Autodesk Fusion 360 part; units mm, degrees
sketch "Sketch1" plane through (0, 0, 0) normal (1, 0, 0) x (0, 1, 0)
  line L0 (0, 0) -> (0, 21)
  line L1 (0, 21) -> (5, 21)
  line L2 (5, 21) -> (5, 8)
  line L3 (5, 8) -> (35, 8)
  line L4 (35, 8) -> (35, 21)
  line L5 (35, 21) -> (40, 21)
  line L6 (40, 21) -> (40, 0)
  line L7 (40, 0) -> (0, 0)
  line L8 (20, 8) -> (20, 0) construction
  dimension "d1" = 8
  dimension "d2" = 30
  dimension "d3" = 5
  dimension "d5" = 5
  dimension "d6" = 13
  dimension "d7" = 13
extrude "Extrude1" add sketch "Sketch1" along normal blind 70
fillet "Fillet1" radius 2.5 2 edges at (35, 40, 21) (35, 0, 21)
sketch "Sketch2" plane through (0, 0, 8) normal (0, 0, 1) x (-1, 0, 0)
  line L0 (0, -35) -> (0, -5)
  line L1 (0, -5) -> (-70, -5)
  line L2 (-70, -5) -> (-70, -35)
  line L3 (-70, -35) -> (0, -35)
  line L4 (0, -5) -> (-70, -5)
  line L5 (-70, -35) -> (-70, -5)
  line L6 (0, -5) -> (0, -35)
  line L7 (0, -35) -> (-70, -35)
  line L8 (-35, -35) -> (-35, -5) construction
  line L9 (-65, -10) -> (-65, -30) construction
  line L10 (-65, -30) -> (-5, -30) construction
  line L11 (-5, -30) -> (-5, -10) construction
  line L12 (-5, -10) -> (-65, -10) construction
  line L13 (-5, -20) -> (-65, -20) construction
  line L14 (-5, -27) -> (-65, -27)
  arc A0 (-65, -27) -> (-65, -32) centre (-65, -29.5) ccw
  line L15 (-65, -32) -> (-5, -32)
  arc A1 (-5, -32) -> (-5, -27) centre (-5, -29.5) ccw
  line L16 (-5, -29.5) -> (-65, -29.5) construction
  line L17 (-65, -22.5) -> (-5, -22.5)
  arc A2 (-5, -22.5) -> (-5, -17.5) centre (-5, -20) ccw
  line L18 (-5, -17.5) -> (-65, -17.5)
  arc A3 (-65, -17.5) -> (-65, -22.5) centre (-65, -20) ccw
  line L19 (-65, -13) -> (-5, -13)
  arc A4 (-5, -13) -> (-5, -8) centre (-5, -10.5) ccw
  line L20 (-5, -8) -> (-65, -8)
  arc A5 (-65, -8) -> (-65, -13) centre (-65, -10.5) ccw
  dimension "d12" = -5
  dimension "d15" = 3
  dimension "d16" = 5
  dimension "d19" = 0
  dimension "d20" = 19
extrude "Extrude2" cut sketch "Sketch2" against normal up to surface (8 mm away) contours L14 A0 L15 A1 | L17 A2 L18 A3 | L19 A4 L20 A5
sketch "Sketch3" plane through (0, 0, 0) normal (0, -1, 0) x (1, 0, 0)
  line L0 (70, 18.5) -> (0, 18.5)
  line L1 (0, 18.5) -> (0, 0)
  line L2 (0, 0) -> (70, 0)
  line L3 (70, 0) -> (70, 18.5)
  line L4 (0, 8) -> (70, 8)
  line L5 (0, 21) -> (70, 21)
  line L6 (0, 21) -> (0, 8)
  line L7 (70, 8) -> (70, 21)
  line L8 (0, 18.5) -> (70, 18.5)
  line L9 (5.5, 10.5) -> (64.5, 10.5)
  arc A0 (64.5, 10.5) -> (64.5, 15.5) centre (64.5, 13) ccw
  line L10 (64.5, 15.5) -> (5.5, 15.5)
  arc A1 (5.5, 15.5) -> (5.5, 10.5) centre (5.5, 13) ccw
  line L11 (5.5, 13) -> (64.5, 13) construction
  dimension "d23" = 5
  dimension "d24" = 3
  dimension "d25" = 3
  dimension "d26" = 3
extrude "Extrude3" cut sketch "Sketch3" against normal up to surface (40 mm away) contours L9 A0 L10 A1
fillet "Fillet2" radius 5 2 edges at (35, 40, 0) (35, 0, 0)
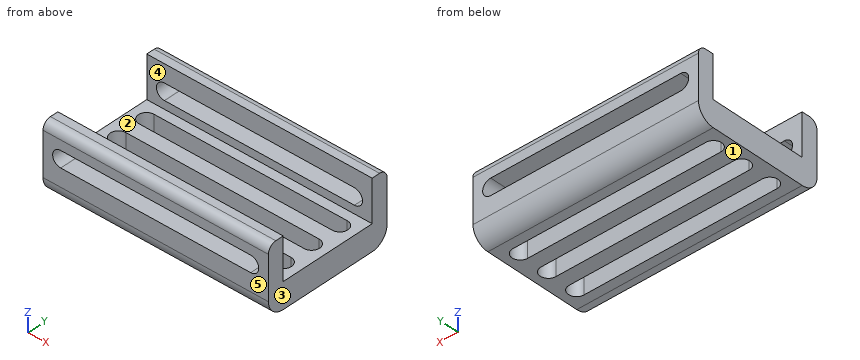
Could you check a few things on this model? Use its own coordinates, in mm. Face numbers are marked on the shaded views. A direction names the side the tool comes from. Coordinates: 2 decimals unless noted, no trailing zeros. Order: outer loops, then holes, each group sorted by start corner. A loop starts at its lowest first (then second) coordinate and runs counter-clockwise, first axis right, second up. Notation, with made-up numbers: (-11.5, -36.75) -> (30.5, -36.75) arc R20 cw to (30.5, -24.75) -> close; hole circle Ø6 at (3.25, 58.5). An arc over 180 degrees is marked (long way). One line per question, with ' | ' between items.
Q1. If I drill on L1, parallel to Y at x = 34.5, z = 5.25; L2, parallel to Y at x = 4.5, z = 10.5; L3, parallel to Y at x = 66.5, z = 4.75, over which ranges is the centre line in solid material (lowest first)?
Return value:
L1: 0 to 8, 13 to 17.5, 22.5 to 27, 32 to 40 | L2: 0 to 5, 35 to 40 | L3: 0.01 to 8.5, 12.5 to 18, 22 to 27.5, 31.5 to 39.99
Q2. I'm going to push flat-ended pins straight in: P1, Ø1, axis at x = 35.5, y = 21, coming from the +Z side; P2, Ø2.5, axis at x = 45.5, y = 36.5, coming from the -Z side; P3, Ø4, axis at x = 33.5, z = 2.5, coming from the -Y side; P4, Ø1.5, axis at x = 24, y = 1.5, coming from the -Z side. Where does each tip first touch, or does it pass through?
Return value:
P1: through | P2: z = 0.01 | P3: y = 0.03 | P4: z = 0.82
Q3. On a 3-axis mill with a long thin cutter (end or side, diameter ignored), from which of +Z, -Z, +X, -X, +Y, -Y can I reach the whole of each face in a straight line? I mean the marked faces 1 and 2. Say none if no direction works.
Return value:
face 1: -Z, +X, -X, +Y, -Y | face 2: +Z, +X, -X
Q4. Imagine slicing it at A-A on z = 13. Please give me the cut outline in (x, y), and give its area (3 significant figures).
Return value:
outline: (0, 0) -> (3, 0) -> (3, 5) -> (0, 5) -> close; (0, 35) -> (3, 35) -> (3, 40) -> (0, 40) -> close; (67, 0) -> (70, 0) -> (70, 5) -> (67, 5) -> close; (67, 35) -> (70, 35) -> (70, 40) -> (67, 40) -> close | area: 60.0 mm²
Q5. Imagine slicing it at D-D on z = 16.5. Please give me the cut outline in (x, y), and give its area (3 significant figures).
Return value:
outline: (0, 0) -> (70, 0) -> (70, 5) -> (0, 5) -> close; (0, 35) -> (70, 35) -> (70, 40) -> (0, 40) -> close | area: 700 mm²
Q6. Thinking about a two-plate mould opening in Y: for the marked faces 3, 4 and 5, which applies, pulls with the +Y half, pulls with the -Y half, needs draft (parallel to the pull), parting line crosses it, or undercut?
Return value:
face 3: needs draft | face 4: undercut | face 5: pulls with the -Y half
Q7. Imagine slicing it at C-C on x = 21. State how many separate pieces and enclosed holes the cut face has, and give its area (3 significant figures).
Return value:
separate pieces: 6 | enclosed holes: 0 | area: 267 mm²
Q8. Imagine slicing it at B-B on y = 12. Please give me the cut outline in (x, z).
Return value:
outline: (0, 0) -> (3, 0) -> (3, 8) -> (0, 8) -> close; (67, 0) -> (70, 0) -> (70, 8) -> (67, 8) -> close
